Can you work these out from the model? Positions are in its coordinate system, mm. Face numbers are marked on the shaded views. A direction names the side the tool comes from. Round coordinates to 2 decimals unless told otherwise and drop trailing zeros. Order: outer loops, then holes, each group sorted by start corner. A loop starts at its lowest first (then second) coordinate and runs counter-clockwise, first axis right, second up. Notation, with made-up numbers: (76.5, -22) -> (81.5, -22) arc R32 ccw to (81.5, 9) -> close; hole circle Ø10 at (-28, -24.75). An arc over 180 degrees is marked (long way). One line per item, written item: value.
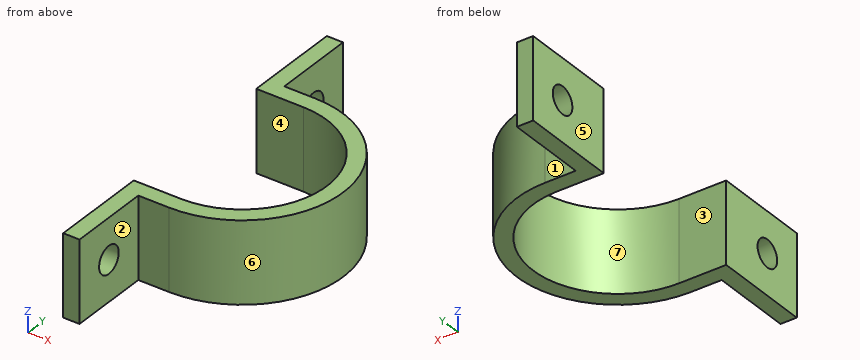
Autodesk Inventor part; units mm, degrees
ref_plane "YZ Plane" through (0, 0, 0) normal (1, 0, 0) x (0, 1, 0)
ref_plane "XZ Plane" through (0, 0, 0) normal (0, 1, 0) x (-1, 0, 0)
ref_plane "XY Plane" through (0, 0, 0) normal (0, 0, 1) x (1, 0, 0)
sketch "Skizze1" plane through (0, 0, 0) normal (0, 0, 1) x (1, 0, 0)
  arc A0 (-12.5, -6) -> (0, 6.5) centre (0, -6) ccw
  arc A1 (0, 6.5) -> (-12.5, -6) centre (0, -6) ccw
  line L0 (-14.35, -116) -> (-14.35, 104)
  line L1 (-6.95, -18.5) -> (0, -18.5)
  arc A2 (0, -18.5) -> (0, 6.5) centre (0, -6) ccw
  line L2 (0, 6.5) -> (-6.95, 6.5)
  line L3 (-6.95, 6.5) -> (-6.95, 20.9)
  line L4 (-6.95, 20.9) -> (-4.55, 20.9)
  line L5 (-4.55, 20.9) -> (-4.55, 8.9)
  line L6 (-4.55, 8.9) -> (0, 8.9)
  arc A3 (0, -20.9) -> (0, 8.9) centre (0, -6) ccw
  line L7 (0, -20.9) -> (-4.55, -20.9)
  line L8 (-4.55, -20.9) -> (-4.55, -32.9)
  line L9 (-4.55, -32.9) -> (-6.95, -32.9)
  line L10 (-6.95, -32.9) -> (-6.95, -18.5)
  point P0 (0, 0)
  point P1 (-14.35, 20.9)
  point P2 (-14.35, 6.5)
  point P3 (0, 6.5)
  point P4 (0, -18.5)
  point P5 (-14.35, -18.5)
  point P6 (-14.35, -32.9)
  dimension "d0" = 2.4
  dimension "d1" = 2.4
  dimension "d2" = 2.4
  dimension "d4" = 12.5
  dimension "d5" = 7.4
  dimension "d7" = 12.5
  dimension "d8" = 12
extrude "Extrusion1" add sketch "Skizze1" against normal blind 12 contours A0 L2 L3 L4 L5 L6 A3 L7 L8 L9 L10 L1
sketch "Skizze2" plane through (-4.55, 8.9, 0) normal (1, 0, 0) x (0, 0, -1)
  line L0 (0, 0) -> (12, 0)
  line L1 (12, -2.4) -> (12, 12)
  line L2 (0, 0) -> (12, 12) construction
  circle A0 centre (6, 6) radius 2
  line L3 (12, -41.8) -> (12, -27.4) construction
  line L4 (12, -41.8) -> (0, -29.8) construction
  line L5 (0, -27.4) -> (0, -41.8) construction
  circle A1 centre (6, -35.8) radius 2
  point P0 (0, -8.9)
  dimension "d11" = 4
extrude "Extrusion2" cut sketch "Skizze2" against normal through all
equation "\"d1\" = d0"
equation "\"d2\" = d0"
equation "\"d7\" = d4"
equation "\"d9\" = d8"
properties part number "12_Motor_Fixation"
Q1. On a 3-axis mill with a long thin cutter (end or side, diameter ignored), from which of +Z, -Z, +X, -X, +Y, -Y can I reach the whole of each face in a straight line? I mean the marked faces 1, 2 and 3. Say none if no direction works.
Answers below:
face 1: +Z, -Z, +X, +Y
face 2: +Z, -Z, +X, -Y
face 3: +Z, -Z, -X
Q2. I want a section at B-B on z = -6. List the corners of the cut face in (x, y) for me, plus the area to 3 significant figures.
Answers below:
outline: (-6.95, -32.9) -> (-4.55, -32.9) -> (-4.55, -28.9) -> (-6.95, -28.9) -> close; (-6.95, -24.9) -> (-4.55, -24.9) -> (-4.55, -20.9) -> (0, -20.9) arc R14.9 ccw to (0, 8.9) -> (-4.55, 8.9) -> (-4.55, 12.9) -> (-6.95, 12.9) -> (-6.95, 6.5) -> (0, 6.5) arc R12.5 cw to (0, -18.5) -> (-6.95, -18.5) -> close; (-6.95, 16.9) -> (-4.55, 16.9) -> (-4.55, 20.9) -> (-6.95, 20.9) -> close
area: 175 mm^2
Q3. I want a section at D-D on z = -2. List the corners of the cut face in (x, y) for me.
Answers below:
outline: (-6.95, -32.9) -> (-4.55, -32.9) -> (-4.55, -20.9) -> (0, -20.9) arc R14.9 ccw to (0, 8.9) -> (-4.55, 8.9) -> (-4.55, 20.9) -> (-6.95, 20.9) -> (-6.95, 6.5) -> (0, 6.5) arc R12.5 cw to (0, -18.5) -> (-6.95, -18.5) -> close
Q4. I want a section at A-A on y = -26.9. List the corners of the cut face in (x, z) for me.
Answers below:
outline: (-6.95, -12) -> (-4.55, -12) -> (-4.55, -8) -> (-6.95, -8) -> close; (-6.95, -4) -> (-4.55, -4) -> (-4.55, 0) -> (-6.95, 0) -> close
Q5. I want a section at C-C on x = 8.5. List the corners of the cut face in (y, z) for me.
Answers below:
outline: (-18.24, -12) -> (-15.17, -12) -> (-15.17, 0) -> (-18.24, 0) -> close; (3.17, -12) -> (6.24, -12) -> (6.24, 0) -> (3.17, 0) -> close
Q6. We'd pull the mould along Y, two halves only. Please class the marked faces 4, 5, 6 and 7: released by +Y, released by -Y, zero draft, split by the parting line, or undercut.
Answers below:
face 4: undercut
face 5: zero draft
face 6: split by the parting line
face 7: undercut
Q7. Please list where these lines run through material, in increasing order: line 1 along Y through (x, z) = (-5.55, -6); line 2 along Y through (x, z) = (-6, -2.75); line 3 along Y through (x, z) = (-4.5, -4).
Answers below:
line 1: -32.9 to -28.9, -24.9 to -18.5, 6.5 to 12.9, 16.9 to 20.9
line 2: -32.9 to -18.5, 6.5 to 20.9
line 3: -20.9 to -18.5, 6.5 to 8.9
Q8. Will these pins go through, and if not, where does the flat tip stop? pin 1 Ø3.5 at (x, z) = (-3, -5) entering from +Y; pin 2 Ø3.5 at (y, z) = (-25, -8.5) entering from +X; pin 3 Ø2 at (x, z) = (3.5, -7.5) entering from +Y; pin 4 Ø5 at (y, z) = (7.5, -2.5) entering from +X.
Answers below:
pin 1: y = 20.9
pin 2: x = -4.55
pin 3: y = 8.69
pin 4: x = 10.05
